Could you check a few things on this model? Use its own coordinates, in mm. Face numbers are marked on the shaded views. A direction names the side the tool comes from. Coordinates: 2 decimals unless noted, no trailing zeros. Write each loop counter-clockwise with the first axis right and the second up, starting at its lowest first coordinate (ties: lowest second). Pieces come first, ordered by that corner, then holes. Notation, with made-up numbers: M -6.75,4.5 L 31.25,4.5 A25 ccw 31.25,26.5 Z; hole C 30.5,32 d2. An arc over 180 degrees is marked long. Answer as CSV lines item,"result". Start each with the question number.
Item 1: If I drill on line 1 along Y through (x, z) = (26.35, 7.25) (3 decimals); line 2 along Z through (x, y) = (0, 27.15), over which ranges is the centre line in solid material (lowest first)? Write a range as [from, to].
Item 2: On a 3-axis mill with a long thin cutter (end or side, diameter ignored), from which of +Z, -Z, +X, -X, +Y, -Y can I reach the whole of each face in a straight line? I mean the marked faces 1, 2, 3, 4 and 5. Say none if no direction works.
Item 3: Suppose I cut it at C-C, the plane z = 7.25. Write out the boundary of the cut face in (x, y) (3 decimals).
Item 4: Suppose I cut it at D-D, the plane y = 26. Write out the boundary of the cut face in (x, z) (3 decimals), and give its area (3 significant figures).
Item 5: I'm going to push flat-ended pins straight in: P1, Ø3, axis at y = 0, z = 7.25, coming from the +X side; P2, Ø4, axis at x = 11.5, z = 8.5, coming from the -Y side; P3, Ø2, axis at y = 8.5, z = 6.5, coming from the +X side; P4, Ø8, axis at y = 12.5, z = 11, coming from the +X side. Where does each tip first touch, or does it pass through?
Item 6: Suppose I cut it at A-A, the plane y = 0. Write out the boundary of the cut face in (x, z), and give its area (3 significant figures).
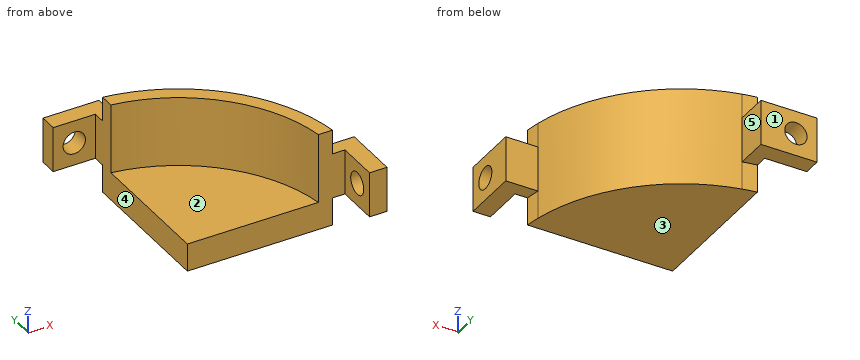
```python
from build123d import *

# Parameters (mm, degrees)
BOSS_EXTRUDE1_DEPTH   = 14.5
M3_CLEARANCE_HOLE1_D  = 3.2
M3_CLEARANCE_HOLE2_D  = 3.2
SKETCH6_W             = 6.05
SKETCH6_H             = 4
CUT_EXTRUDE1_DEPTH    = 10
SKETCH7_W             = 4
SKETCH7_H             = 6.05
CUT_EXTRUDE2_DEPTH    = 10
BOSS_EXTRUDE7_DEPTH   = 14
SKETCH14_W            = 57.002666796
SKETCH14_H            = 41.192482136
CUT_EXTRUDE4_DEPTH    = 15
CUT_EXTRUDE5_DEPTH    = 10
CUT_EXTRUDE8_DEPTH    = 20
CUT_EXTRUDE9_DEPTH    = 4
CUT_EXTRUDE9_START    = 10.5
CUT_EXTRUDE9_2_DEPTH  = 3.5
CUT_EXTRUDE10_DEPTH   = 4
CUT_EXTRUDE10_START   = 10.5
CUT_EXTRUDE10_2_DEPTH = 3.5


# Read off the part's stored shape, not the designer's step: Cut-Extrude9, Cut-Extrude10
with BuildPart() as part:
    # Sketch1 → Boss-Extrude1 (new body)
    with BuildSketch(Plane.XY):
        with BuildLine():
            Line((3.025, 25.6), (-3.025, 25.6))
            Line((-3.025, 25.6), (-3.025, 28.1))
            Line((-3.025, 28.1), (3.025, 28.1))
            ThreePointArc((3.025, 28.1), (21.312111091, 21.312111091), (28.1, 3.025))
            Line((28.1, 3.025), (28.1, -3.025))
            Line((28.1, -3.025), (25.6, -3.025))
            Line((25.6, -3.025), (25.6, 3.025))
            ThreePointArc((25.6, 3.025), (18.987935585, 18.987935585), (3.025, 25.6))
        make_face()
    extrude(amount=BOSS_EXTRUDE1_DEPTH)

    # M3 Clearance Hole1 (through all)
    with Locations(Plane(origin=(0, 28.1, 0), x_dir=(1, 0, 0), z_dir=(0, 1, 0))):
        with Locations((0, -7.25)):
            Hole(M3_CLEARANCE_HOLE1_D / 2)

    # M3 Clearance Hole2 (through all)
    with Locations(Plane(origin=(28.1, 0, 0), x_dir=(0, 0, -1), z_dir=(1, 0, 0))):
        with Locations((-7.25, 0)):
            Hole(M3_CLEARANCE_HOLE2_D / 2)

    # Sketch6 → Cut-Extrude1 (cut)
    with BuildSketch(Plane(origin=(0, 28.1, 0), x_dir=(1, 0, 0), z_dir=(0, 1, 0))):
        with Locations((0, -12.5)):
            Rectangle(SKETCH6_W, SKETCH6_H)
        with Locations((0, -2)):
            Rectangle(SKETCH6_W, SKETCH6_H)
    extrude(amount=-CUT_EXTRUDE1_DEPTH, mode=Mode.SUBTRACT)

    # Sketch7 → Cut-Extrude2 (cut)
    with BuildSketch(Plane(origin=(28.1, 0, 0), x_dir=(0, 0, -1), z_dir=(1, 0, 0))):
        with Locations((-12.5, 0)):
            Rectangle(SKETCH7_W, SKETCH7_H)
        with Locations((-2, 0)):
            Rectangle(SKETCH7_W, SKETCH7_H)
    extrude(amount=-CUT_EXTRUDE2_DEPTH, mode=Mode.SUBTRACT)

    # Sketch8 → Boss-Extrude7 (add)
    with BuildSketch(Plane(origin=(0, 0, 0), x_dir=(-1, 0, 0), z_dir=(0, 0, -1))):
        with BuildLine():
            Line((-31.03541973, 3.015), (-3.015, 3.015))
            Line((-3.015, 3.015), (-3.015, 31.03541973))
            ThreePointArc((-3.015, 31.03541973), (-22.048667792, 22.048667792), (-31.03541973, 3.015))
        make_face()
    extrude(amount=-BOSS_EXTRUDE7_DEPTH)

    # Sketch14 → Cut-Extrude4 (cut)
    with BuildSketch(Plane.XY.offset(14)):
        with Locations((13.446699297, 19.415661607)):
            Rectangle(SKETCH14_W, SKETCH14_H)
    extrude(amount=CUT_EXTRUDE4_DEPTH, mode=Mode.SUBTRACT)

    # Sketch15 → Cut-Extrude5 (cut)
    with BuildSketch(Plane.XY.offset(14)):
        with BuildLine():
            Line((3.015, 21.792424716), (3.015, 3.015))
            Line((3.015, 3.015), (21.792424716, 3.015))
            ThreePointArc((21.792424716, 3.015), (15.556349186, 15.556349186), (3.015, 21.792424716))
        make_face()
    extrude(amount=-CUT_EXTRUDE5_DEPTH, mode=Mode.SUBTRACT)

    # Sketch16 → Cut-Extrude8 (cut)
    with BuildSketch(Plane.XY.offset(14)):
        with BuildLine():
            Line((5.015, 23.47018907), (5.015, 28.1))
            Line((5.015, 28.1), (3.015, 28.1))
            Line((3.015, 28.1), (3.015, 36.20716296))
            Line((3.015, 36.20716296), (34.30048071, 28.1))
            Line((34.30048071, 28.1), (32.410436515, 3.015))
            Line((32.410436515, 3.015), (28.1, 3.015))
            Line((28.1, 3.015), (28.1, 5.015))
            Line((28.1, 5.015), (23.47018907, 5.015))
            ThreePointArc((23.47018907, 5.015), (16.970562748, 16.970562748), (5.015, 23.47018907))
        make_face()
    extrude(amount=-CUT_EXTRUDE8_DEPTH, mode=Mode.SUBTRACT)

    # Cut-Extrude9 outline → Cut-Extrude9 (cut)
    with BuildSketch(Plane.XY):
        with BuildLine():
            Line((28.1, 3.015), (28.1, 5.015))
            Line((28.1, 5.015), (23.47018907, 5.015))
            ThreePointArc((23.47018907, 5.015), (23.661169237, 4.018590587), (23.809867177, 3.015))
            Line((23.809867177, 3.015), (28.1, 3.015))
        make_face()
    extrude(amount=CUT_EXTRUDE9_DEPTH, mode=Mode.SUBTRACT)

    # Cut-Extrude9 2 outline → Cut-Extrude9 2 (cut)
    with BuildSketch(Plane.XY.offset(CUT_EXTRUDE9_START)):
        with BuildLine():
            Line((28.1, 3.015), (28.1, 5.015))
            Line((28.1, 5.015), (23.47018907, 5.015))
            ThreePointArc((23.47018907, 5.015), (23.661169237, 4.018590587), (23.809867177, 3.015))
            Line((23.809867177, 3.015), (28.1, 3.015))
        make_face()
    extrude(amount=CUT_EXTRUDE9_2_DEPTH, mode=Mode.SUBTRACT)

    # Cut-Extrude10 outline → Cut-Extrude10 (cut)
    with BuildSketch(Plane.XY):
        with BuildLine():
            Line((5.015, 28.1), (3.015, 28.1))
            Line((3.015, 28.1), (3.015, 23.809867177))
            ThreePointArc((3.015, 23.809867177), (4.018590587, 23.661169237), (5.015, 23.47018907))
            Line((5.015, 23.47018907), (5.015, 28.1))
        make_face()
    extrude(amount=CUT_EXTRUDE10_DEPTH, mode=Mode.SUBTRACT)

    # Cut-Extrude10 2 outline → Cut-Extrude10 2 (cut)
    with BuildSketch(Plane.XY.offset(CUT_EXTRUDE10_START)):
        with BuildLine():
            Line((5.015, 28.1), (3.015, 28.1))
            Line((3.015, 28.1), (3.015, 23.809867177))
            ThreePointArc((3.015, 23.809867177), (4.018590587, 23.661169237), (5.015, 23.47018907))
            Line((5.015, 23.47018907), (5.015, 28.1))
        make_face()
    extrude(amount=CUT_EXTRUDE10_2_DEPTH, mode=Mode.SUBTRACT)


solid = part.part
```
Ans:
1,line 1,"y = [-3.025, -1.6], [1.6, 5.015]"
1,line 2,"z = [4, 5.65], [8.85, 10.5]"
2,face 1,"+Z, -Z, +X, -X, +Y"
2,face 2,"+Z, -X, -Y"
2,face 3,"-Z, +X, -X, +Y, -Y"
2,face 4,"+Z, -Z, -X, -Y"
2,face 5,"+Z, -Z, +X, +Y"
3,outline,"M -3.025,25.6 L -1.6,25.6 L -1.6,28.1 L -3.025,28.1 Z; M 1.6,25.6 L 3.015,25.6 L 3.015,21.792 A22 cw 21.792,3.015 L 25.6,3.015 L 25.6,1.6 L 28.1,1.6 L 28.1,5.015 L 23.47,5.015 A24 ccw 5.015,23.47 L 5.015,28.1 L 1.6,28.1 Z; M 25.6,-3.025 L 28.1,-3.025 L 28.1,-1.6 L 25.6,-1.6 Z"
4,outline,"M -3.025,4 L 5.015,4 L 5.015,10.5 L -3.025,10.5 Z; hole C 0,7.25 d3.2"
4,area,"44.2 mm^2"
5,P1,"passes through"
5,P2,"stops at y = 17.37"
5,P3,"stops at x = 22.8"
5,P4,"stops at x = 22.44"
6,outline,"M 25.6,4 L 28.1,4 L 28.1,5.65 L 25.6,5.65 Z; M 25.6,8.85 L 28.1,8.85 L 28.1,10.5 L 25.6,10.5 Z"
6,area,"8.25 mm^2"
